For this review, use the dimensioned drawing (mm, ordinates from the lowest corner) and the shaded views. Give positions to 0.01 mm unless a question says otherwise; leave off trailing zeros. Order: outer loops, then holes, each group sorted by start corner. A loop starts at its lowest first (then second) coordinate and runs counter-clockwise, first axis right, second up. Notation, with made-up numbers: (86, -2) -> (139, -2) arc R9 ccw to (139, 5) -> close; hole circle Ø3 at (-37.75, 77). An arc over 180 degrees is marked (long way). One line per item, written item: value. Start each with the question number.
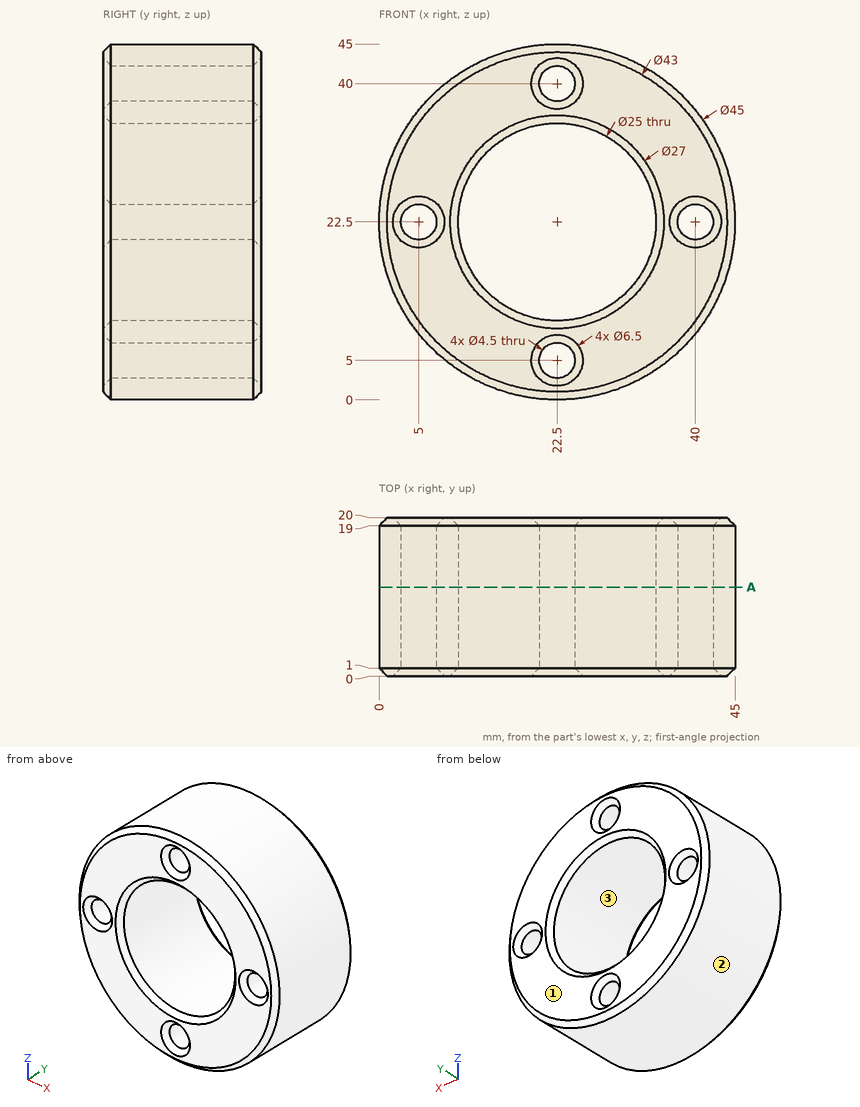
Q1. For pin 1 Ø1 at (x, y) = (33.5, 9.5) entering from -Z; pin 2 Ø3 at (x, y) = (28, 12) entering from -Z; pin 3 Ø4 at (y, z) = (7.5, 20.5) entering from +X, all flat-tipped, find the tip position at first contact; note any pin that passes through.
Q2. Take a section at A-A (y = 11.25). State the section outline as (x, z) points.
Q3. Mouldability with a two-part tool opening along Z and no side actions: class the marked faces 1, 2 and 3 as pulls with the +Z half, pulls with the -Z half, needs draft (parallel to the pull), parting line crosses it, or undercut.
Q4. For line 1 along X through (y, z) = (14.5, 22.5); line 2 along Z through (x, y) = (24.5, 12.75); line 3 along Z through (x, y) = (22, 9), list the stretches that pass through material, from the lowest coordinate up.
Answers below:
1. pin 1: stops at z = 2.6
1. pin 2: stops at z = 0.36
1. pin 3: stops at x = 45
2. outline: circle Ø45 at (22.5, 22.5); hole circle Ø4.5 at (5, 22.5); hole circle Ø25 at (22.5, 22.5); hole circle Ø4.5 at (22.5, 5); hole circle Ø4.5 at (22.5, 40); hole circle Ø4.5 at (40, 22.5)
3. face 1: needs draft
3. face 2: parting line crosses it
3. face 3: undercut
4. line 1: x = 0 to 2.75, 7.25 to 10, 35 to 37.75, 42.25 to 45
4. line 2: z = 0.09 to 3.97, 6.03 to 10.16, 34.84 to 38.97, 41.03 to 44.91
4. line 3: z = 0.01 to 2.81, 7.19 to 10.01, 34.99 to 37.81, 42.19 to 44.99
